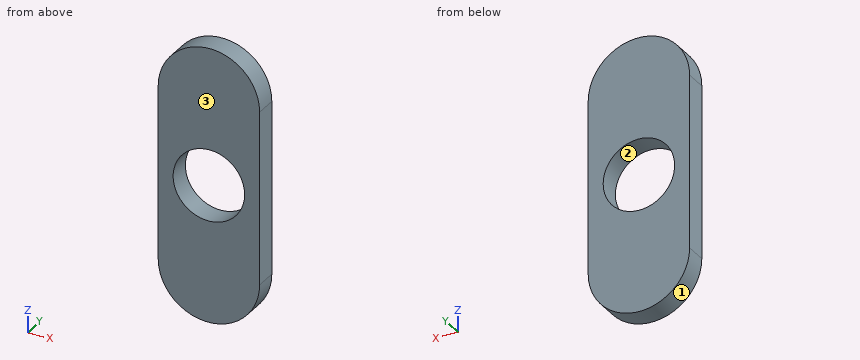
```python
from build123d import *

# Parameters (mm, degrees)
F0_R     = 13.25
F0_R_2   = 11.1
F1_DEPTH = 3.5
F2_START = 2.5
F2_DEPTH = 1
F3_START = -2.5
F3_DEPTH = 1


with BuildPart() as f1:
    # F0 (on Front) → F1 (new body, symmetric)
    with BuildSketch(Plane.XZ):
        with BuildLine():
            Line((15.75, -26.85), (15.75, 26.85))
            ThreePointArc((15.75, 26.85), (0, 42.6), (-15.75, 26.85))
            Line((-15.75, 26.85), (-15.75, -26.85))
            ThreePointArc((-15.75, -26.85), (0, -42.6), (15.75, -26.85))
        make_face()
        with Locations((0, -26.85)):
            Circle(F0_R, mode=Mode.SUBTRACT)
        Circle(F0_R_2, mode=Mode.SUBTRACT)
        with Locations((0, 26.85)):
            Circle(F0_R, mode=Mode.SUBTRACT)
    extrude(amount=F1_DEPTH, both=True)

    # F0 (on Front) → F2 (join)
    with BuildSketch(Plane.XZ.offset(F2_START)):
        with Locations((0, 26.85)):
            Circle(F0_R)
        with Locations((0, -26.85)):
            Circle(F0_R)
    extrude(amount=F2_DEPTH)

    # F0 (on Front) → F3 (join)
    with BuildSketch(Plane.XZ.offset(F3_START)):
        with Locations((0, 26.85)):
            Circle(F0_R)
        with Locations((0, -26.85)):
            Circle(F0_R)
    extrude(amount=-F3_DEPTH)


solid = f1.part
```
Model file for the job. Use its own axes, mm. Face numbers are marked on the shaded views. Round coordinates to 2 decimals unless told otherwise and drop trailing zeros. Write each loop counter-clockwise with the first axis right and the second up, starting at its lowest first coordinate (ties: lowest second). Pieces come first, ordered by that corner, then holes. Notation, with made-up numbers: (7.5, 55.5) - (28.5, 55.5) arc R26 cw to (28.5, 75.5) - close; hole circle Ø10 at (45.5, 81.5). An arc over 180 degrees is marked (long way). One line per item, written item: value.
(1) Two-plate mould, pull along Z, no slides. Class the marked faces 1, 2 and 3: pulls with the +Z half, pulls with the -Z half, needs draft (parallel to the pull), parting line crosses it, or undercut.
Values follow:
face 1: pulls with the -Z half
face 2: undercut
face 3: needs draft
(2) Drop a flat-ended pin along its axis: P1, Ø4, axis at x = -7.5, y = 0.5, coming from the -Z side. Give the stop position or say it passes through.
Values follow:
P1: stops at z = -41.61
(3) Cut at C-C, the plane z = 0. Give the cut face in (x, y), plus the area to 3 significant figures.
Values follow:
outline: (-15.75, -3.5) - (-11.1, -3.5) - (-11.1, 3.5) - (-15.75, 3.5) - close; (11.1, -3.5) - (15.75, -3.5) - (15.75, 3.5) - (11.1, 3.5) - close
area: 65.1 mm²
(4) Wall check: probe 1 along Z at (x, y) = (0, -0.25); probe 2 along Y at (x, z) = (0, 36); probe 3 along Z at (x, y) = (-3.5, -1.25). Give the ranges that are in metal, low to high.
Values follow:
probe 1: z = -42.6 to -40.1, -13.6 to -11.1, 11.1 to 13.6, 40.1 to 42.6
probe 2: y = -3.5 to -2.5, 2.5 to 3.5
probe 3: z = -42.21 to -39.63, -14.07 to -10.53, 10.53 to 14.07, 39.63 to 42.21
(5) Cut at B-B, the plane y = 0. Give the cut face in (x, z).
Values follow:
outline: (-15.75, -26.85) arc R15.75 ccw to (15.75, -26.85) - (15.75, 26.85) arc R15.75 ccw to (-15.75, 26.85) - close; hole circle Ø26.5 at (0, -26.85); hole circle Ø26.5 at (0, 26.85); hole circle Ø22.2 at (0, 0)
(6) Cut at D-D, the plane x = -6. Give the cut face in (y, z).
Values follow:
outline: (-3.5, -41.41) - (3.5, -41.41) - (3.5, -9.34) - (-3.5, -9.34) - close; (-3.5, 9.34) - (3.5, 9.34) - (3.5, 41.41) - (-3.5, 41.41) - close; hole (-2.5, -38.66) - (2.5, -38.66) - (2.5, -15.04) - (-2.5, -15.04) - close; hole (-2.5, 15.04) - (2.5, 15.04) - (2.5, 38.66) - (-2.5, 38.66) - close
(7) Cut at A-A, the plane x = 0. Give the cut face in (y, z), plus the area to 3 significant figures.
Values follow:
outline: (-3.5, -42.6) - (3.5, -42.6) - (3.5, -11.1) - (-3.5, -11.1) - close; (-3.5, 11.1) - (3.5, 11.1) - (3.5, 42.6) - (-3.5, 42.6) - close; hole (-2.5, -40.1) - (2.5, -40.1) - (2.5, -13.6) - (-2.5, -13.6) - close; hole (-2.5, 13.6) - (2.5, 13.6) - (2.5, 40.1) - (-2.5, 40.1) - close
area: 176 mm²
